from build123d import *

# Parameters (mm, degrees)
CROQUIS1_R              = 1
SALIENTE_EXTRUIR1_DEPTH = 4
CROQUIS5_R              = 1.25
CORTAR_EXTRUIR2_DEPTH   = 6
SALIENTE_EXTRUIR2_START = -4
CROQUIS6_R              = 3
SALIENTE_EXTRUIR2_DEPTH = 4
CROQUIS8_R              = 1.25
CORTAR_EXTRUIR4_DEPTH   = 5
CORTAR_EXTRUIR5_START   = -31.8
CROQUIS8_2_R            = 1.25
CORTAR_EXTRUIR5_DEPTH   = 5
REDONDEO1_R             = 3
REDONDEO2_R             = 1.6
CROQUIS7_R              = 1.6
CORTAR_EXTRUIR3_DEPTH   = 4


with BuildPart() as part:
    # Croquis1 → Saliente-Extruir1 (new body)
    with BuildSketch(Plane.XY):
        with BuildLine():
            Line((12, 0), (12, 18.4))
            Line((12, 18.4), (0, 18.4))
            ThreePointArc((0, 18.4), (-18.4, 0), (0, -18.4))
            Line((0, -18.4), (12, -18.4))
            Line((12, -18.4), (12, 0))
        make_face()
        with Locations((-8, -6.72)):
            Circle(CROQUIS1_R, mode=Mode.SUBTRACT)
        with Locations((-8, 6.72)):
            Circle(CROQUIS1_R, mode=Mode.SUBTRACT)
        with Locations((-5.9, -6.72)):
            Circle(CROQUIS1_R, mode=Mode.SUBTRACT)
        with Locations((-5.9, 6.72)):
            Circle(CROQUIS1_R, mode=Mode.SUBTRACT)
        with Locations((-3.8, -6.72)):
            Circle(CROQUIS1_R, mode=Mode.SUBTRACT)
        with Locations((-3.8, 6.72)):
            Circle(CROQUIS1_R, mode=Mode.SUBTRACT)
        with Locations((-1.7, -6.72)):
            Circle(CROQUIS1_R, mode=Mode.SUBTRACT)
        with Locations((-1.7, 6.72)):
            Circle(CROQUIS1_R, mode=Mode.SUBTRACT)
        with Locations((0.4, -6.72)):
            Circle(CROQUIS1_R, mode=Mode.SUBTRACT)
        with Locations((0.4, 6.72)):
            Circle(CROQUIS1_R, mode=Mode.SUBTRACT)
        with Locations((2.5, -6.72)):
            Circle(CROQUIS1_R, mode=Mode.SUBTRACT)
        with Locations((2.5, 6.72)):
            Circle(CROQUIS1_R, mode=Mode.SUBTRACT)
        with Locations((4.6, -6.72)):
            Circle(CROQUIS1_R, mode=Mode.SUBTRACT)
        with Locations((4.6, 6.72)):
            Circle(CROQUIS1_R, mode=Mode.SUBTRACT)
        with Locations((6.7, -6.72)):
            Circle(CROQUIS1_R, mode=Mode.SUBTRACT)
        with Locations((6.7, 6.72)):
            Circle(CROQUIS1_R, mode=Mode.SUBTRACT)
        with Locations((8.8, -6.72)):
            Circle(CROQUIS1_R, mode=Mode.SUBTRACT)
        with Locations((8.8, 6.72)):
            Circle(CROQUIS1_R, mode=Mode.SUBTRACT)
        with BuildLine():
            Line((7, 3), (-7, 3))
            ThreePointArc((-7, 3), (-10, 0), (-7, -3))
            Line((-7, -3), (7, -3))
            ThreePointArc((7, -3), (10, 0), (7, 3))
        make_face(mode=Mode.SUBTRACT)
    extrude(amount=SALIENTE_EXTRUIR1_DEPTH)

    # Croquis5 → Cortar-Extruir2 (cut)
    with BuildSketch(Plane(origin=(12, 0, 0), x_dir=(0, 0, -1), z_dir=(1, 0, 0))):
        with Locations((-2, 13.4)):
            Circle(CROQUIS5_R)
        with Locations(Location((-2, -13.4, 0), (0, 0, 180))):
            Circle(CROQUIS5_R)
    extrude(amount=-CORTAR_EXTRUIR2_DEPTH, mode=Mode.SUBTRACT)

    # Croquis6 → Saliente-Extruir2 (add)
    with BuildSketch(Plane.XY.offset(4).offset(SALIENTE_EXTRUIR2_START)):
        with BuildLine():
            Line((-31.4, 5), (-31.4, -5))
            Line((-31.4, -5), (-17.707625476, -5))
            ThreePointArc((-17.707625476, -5), (-18.4, 0), (-17.707625476, 5))
            Line((-17.707625476, 5), (-31.4, 5))
        make_face()
        with Locations((-26.4, 0)):
            Circle(CROQUIS6_R, mode=Mode.SUBTRACT)
    extrude(amount=SALIENTE_EXTRUIR2_DEPTH)

    # Croquis8 → Cortar-Extruir4 (cut)
    with BuildSketch(Plane(origin=(0, 18.4, 0), x_dir=(1, 0, 0), z_dir=(0, 1, 0))):
        with Locations(Location((4, -2, 0), (0, 0, 270))):
            Circle(CROQUIS8_R)
    extrude(amount=-CORTAR_EXTRUIR4_DEPTH, mode=Mode.SUBTRACT)

    # Croquis8<2> → Cortar-Extruir5 (cut)
    with BuildSketch(Plane(origin=(0, 18.4, 0), x_dir=(1, 0, 0), z_dir=(0, 1, 0)).offset(CORTAR_EXTRUIR5_START)):
        with Locations(Location((4, -2, 0), (0, 0, 270))):
            Circle(CROQUIS8_2_R)
    extrude(amount=-CORTAR_EXTRUIR5_DEPTH, mode=Mode.SUBTRACT)

    # Redondeo1
    redondeo1_edges = [part.edges().sort_by_distance(p)[0] for p in [
        (-31.4, 5, 2),
        (-31.4, -5, 2),
    ]]
    fillet(redondeo1_edges, radius=REDONDEO1_R)

    # Redondeo2
    redondeo2_edges = [part.edges().sort_by_distance(p)[0] for p in [
        (-17.707625476, 5, 2),
        (-17.707625476, -5, 2),
    ]]
    fillet(redondeo2_edges, radius=REDONDEO2_R)

    # Croquis7 → Cortar-Extruir3 (cut)
    with BuildSketch(Plane.XY.offset(4)):
        with Locations((4, 19.4)):
            Circle(CROQUIS7_R)
        with Locations((4, -19.4)):
            Circle(CROQUIS7_R)
        with Locations((13, 13.4)):
            Circle(CROQUIS7_R)
        with Locations((13, -13.4)):
            Circle(CROQUIS7_R)
    extrude(amount=-CORTAR_EXTRUIR3_DEPTH, mode=Mode.SUBTRACT)


solid = part.part
The listing builds one solid part. Answer for the finished solid, in the listing's coordinates (mm). A direction names the side the tool comes from. Coordinates: 2 decimals unless noted, no trailing zeros. Write each loop counter-clockwise with the first axis right and the second up, starting at its lowest first coordinate (ties: lowest second). Pieces come first, ordered by that corner, then holes. Notation, with made-up numbers: M -8,-17 L 14,-17 A22 ccw 14,22 Z; hole C 19,-5 d1. An arc over 180 degrees is marked long. Put each result on its own line as item: value. Start each with the question number.
1. A cutting plane is placed at A-A on x = -7.5. Write down the section's boundary in (y, z).
2. A cutting plane is placed at B-B on y = -16. Write down the section's boundary in (x, z).
3. For a pull along Z with two mould halves and no side action, classify faces 1 (the flat face through (-5, 4, 4)), 2 (the cylindrical face through (3.521, -15.865, 3.155)), 3 (the flat face through (-5, 4, 0)), 4 (the cylindrical face through (1.763, 7.396, 1.972)) as pulls with the +Z half, pulls with the -Z half, needs draft (parallel to the pull), parting line crosses it, or undercut.
4. A cutting plane is placed at C-C on x = -20.5. Write down the section's boundary in (y, z), then the cut area to 3 significant figures.
5. Consider line 1 (Y direction, x = 0.4, z = 2.8); line 2 (Y direction, x = 4.6, z = 2.95); line 3 (X direction, y = -1.5, z = 3.45). Determine where each line is inside the solid, lowest interval first. Write a range as from..to.
6. Which of the six approach directions +Z, -Z, +X, -X, +Y, -Y give full straight-line access (tool end or side, diameter ignored) to faces 5 (the cylindrical face through (-10, 0, 2)), 6 (the cylindrical face through (9.042, 12.921, 0.845)), 7 (the flat face through (4, 13.4, 2))?
7. Flat-ended cylindrical pins translate along their axes: P1, Ø1.2, axis at x = -25.5, z = 2, coming from the -Y side; P2, Ø1.5, axis at y = -13.5, z = 3, coming from the -X side; P3, Ø1, axis at y = -6.5, z = 2, coming from the -X side. Find the tip coordinate at first contact, or state that the pin passes through.
8. A cutting plane is placed at D-D on y = -6.72. Count the separate pieces of the cut face and the enclosed holes in it, then the cut area to 3 significant figures.
Resolved:
1. outline: M -16.8,0 L -7.59,0 L -7.59,4 L -16.8,4 Z; M -5.85,0 L -2.96,0 L -2.96,4 L -5.85,4 Z; M 2.96,0 L 5.85,0 L 5.85,4 L 2.96,4 Z; M 7.59,0 L 16.8,0 L 16.8,4 L 7.59,4 Z
2. outline: M -9.09,0 L 12,0 L 12,4 L -9.09,4 Z; hole C 4,2 d2.5
3. face 1: pulls with the +Z half
3. face 2: undercut
3. face 3: pulls with the -Z half
3. face 4: needs draft
4. outline: M -5,0 L 5,0 L 5,4 L -5,4 Z
4. area: 40.0 mm2
5. line 1: y = -18.4..-7.72, -5.72..-3, 3..5.72, 7.72..18.4
5. line 2: y = -13.4..-7.72, -5.72..-3, 3..5.72, 7.72..13.4
5. line 3: x = -31.4..-29, -23.8..-9.6, 9.6..12
6. face 5: +Z, -Z
6. face 6: +X
6. face 7: +Y
7. P1: stops at y = -5
7. P2: stops at x = -13.27
7. P3: stops at x = -17.4
8. separate pieces: 10
8. enclosed holes: 0
8. area: 44.5 mm2
